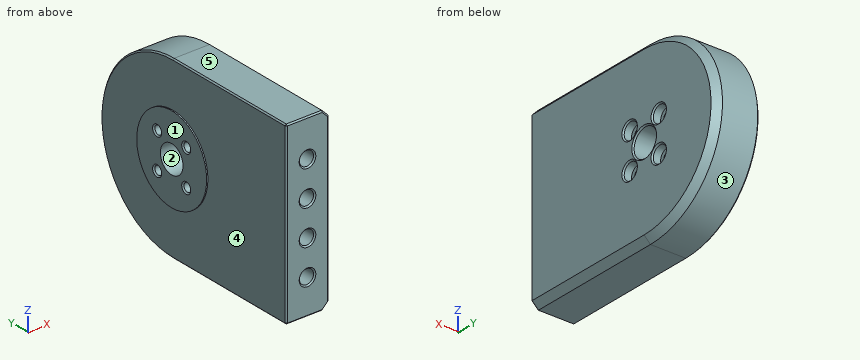
from build123d import *

# Parameters (mm, degrees)
SKETCH1_R                                           = 35
SKETCH1_R_2                                         = 5.5
SKETCH1_R_3                                         = 17
BOSS_EXTRUDE1_DEPTH                                 = 17
BOSS_EXTRUDE2_START                                 = -0.5
SKETCH1_3_R                                         = 17
SKETCH1_3_R_2                                       = 5.5
BOSS_EXTRUDE2_DEPTH                                 = 0.5
CBORE_FOR_M3_HEX_SOCKET_HEAD_CAP_SCREW1_D           = 3.4
CBORE_FOR_M3_HEX_SOCKET_HEAD_CAP_SCREW1_CBORE_D     = 6.5
CBORE_FOR_M3_HEX_SOCKET_HEAD_CAP_SCREW1_CBORE_DEPTH = 3.4
F_5_6_5_6_DIAMETER_HOLE1_D                          = 5.6
F_5_6_5_6_DIAMETER_HOLE1_DEPTH                      = 8
F_5_6_5_6_DIAMETER_HOLE1_TIP                        = 1.682409733
F_2_5MM_CHAMFER1_SIZE                               = 2.5
F_0_5MM_CHAMFER2_SIZE                               = 0.5


with BuildPart() as part:
    # Sketch1 → Boss-Extrude1 (new body)
    # profile 1 of 3: a face of its own
    with BuildSketch(Plane(origin=(0, 0, 0), x_dir=(0, 0, -1), z_dir=(1, 0, 0))):
        Circle(SKETCH1_R)
        Circle(SKETCH1_R_2, mode=Mode.SUBTRACT)
    # profile 2 of 3: a face of its own
    with BuildSketch(Plane(origin=(0, 0, 0), x_dir=(0, 0, -1), z_dir=(1, 0, 0))):
        with BuildLine():
            ThreePointArc((35, 0), (0, -35), (-35, 0))
            Line((-35, 0), (-35, -55))
            Line((-35, -55), (35, -55))
            Line((35, -55), (35, 0))
        make_face()
    # profile 3 of 3: a face of its own
    with BuildSketch(Plane(origin=(0, 0, 0), x_dir=(0, 0, -1), z_dir=(1, 0, 0))):
        Circle(SKETCH1_R_3)
        Circle(SKETCH1_R_2, mode=Mode.SUBTRACT)
    extrude(amount=BOSS_EXTRUDE1_DEPTH)

    # Sketch1<3> → Boss-Extrude2 (add)
    with BuildSketch(Plane(origin=(0, 0, 0), x_dir=(0, 0, -1), z_dir=(1, 0, 0)).offset(BOSS_EXTRUDE2_START)):
        Circle(SKETCH1_3_R)
        Circle(SKETCH1_3_R_2, mode=Mode.SUBTRACT)
    extrude(amount=BOSS_EXTRUDE2_DEPTH)

    # CBORE for M3 Hex Socket Head Cap Screw1 (through all)
    with Locations(Plane(origin=(17, 0, 0), x_dir=(0, 0, -1), z_dir=(1, 0, 0))):
        with Locations((-7.071067812, 7.071067812), (7.071067812, 7.071067812), (7.071067812, -7.071067812), (-7.071067812, -7.071067812)):
            CounterBoreHole(CBORE_FOR_M3_HEX_SOCKET_HEAD_CAP_SCREW1_D / 2, CBORE_FOR_M3_HEX_SOCKET_HEAD_CAP_SCREW1_CBORE_D / 2, CBORE_FOR_M3_HEX_SOCKET_HEAD_CAP_SCREW1_CBORE_DEPTH)

    # Ø5.6 (5.6) Diameter Hole1
    with Locations(Plane(origin=(0, -55, 0), x_dir=(-1, 0, 0), z_dir=(0, -1, 0))):
        with Locations((-8.5, -20.2), (-8.5, 21.2), (-8.5, 7.4), (-8.5, -6.4)):
            Hole(F_5_6_5_6_DIAMETER_HOLE1_D / 2, depth=F_5_6_5_6_DIAMETER_HOLE1_DEPTH)
            with Locations((0, 0, -(F_5_6_5_6_DIAMETER_HOLE1_DEPTH + F_5_6_5_6_DIAMETER_HOLE1_TIP / 2))):  # 118° drill point
                Cone(0, F_5_6_5_6_DIAMETER_HOLE1_D / 2, F_5_6_5_6_DIAMETER_HOLE1_TIP, mode=Mode.SUBTRACT)

    # 2,5mm Chamfer1
    f_2_5mm_chamfer1_edges = [part.edges().sort_by_distance(p)[0] for p in [
        (17, -27.5, 35),
        (17, -27.5, -35),
        (17, 35, 0),
    ]]
    chamfer(f_2_5mm_chamfer1_edges, length=F_2_5MM_CHAMFER1_SIZE)

    # 0,5mm Chamfer2
    f_0_5mm_chamfer2_edges = [part.edges().sort_by_distance(p)[0] for p in [
        (17, 0, 5.5),
        (17, 7.071067812, 10.321067812),
        (-0.5, 7.071067812, 5.371067812),
        (17, -7.071067812, 10.321067812),
        (-0.5, -7.071067812, 5.371067812),
        (17, -7.071067812, -3.821067812),
        (-0.5, -7.071067812, -8.771067812),
        (17, 7.071067812, -3.821067812),
        (-0.5, 7.071067812, -8.771067812),
        (5.7, -55, 20.2),
        (5.7, -55, 6.4),
        (5.7, -55, -7.4),
        (5.7, -55, -21.2),
        (0, -27.5, -35),
        (7.25, -55, -35),
        (17, -55, 0),
        (7.25, -55, 35),
        (0, -55, 0),
        (15.75, -55, 33.75),
        (15.75, -55, -33.75),
        (0, -27.5, 35),
        (0, 35, 0),
    ]]
    chamfer(f_0_5mm_chamfer2_edges, length=F_0_5MM_CHAMFER2_SIZE)


solid = part.part
Check sheet for the modelled part. Datum: model origin and axes. Units: mm. Face numbers are marked on the shaded views. A direction names the side the tool comes from. Give positions to 0.01 mm unless a question says otherwise; leave off trailing zeros. Write each loop counter-clockwise with the first axis right and the second up, starting at its lowest first coordinate (ties: lowest second). Pieces come first, ordered by that corner, then holes. Notation, with made-up numbers: (73, -18.75) -> (117, -18.75) arc R17 ccw to (117, 2.25) -> close; hole circle Ø5 at (-14.5, 58.5). An arc over 180 degrees is marked (long way). One line per item, written item: value. Start each with the question number.
Item 1: Draft check along Y on the marked faces 1, 2 and 3. Enter one of: +Y half, -Y half, draft (parallel to the pull), parting line (faces both ways), or undercut.
Item 2: Gauge pin test, flat ends, axial feed: pin 1 (9 mm diameter, centred on y = 0, z = 0, fed in from -X); pin 2 (5 mm diameter, centred on y = 7, z = 7, fed in from +X); pin 3 (2 mm diameter, centred on y = -13, z = -21, fed in from -X); pin 4 (3.5 mm diameter, centred on x = 8.5, z = 20.2, fed in from -Y). Record the tip position at first contact, or that the pin passes through.
Item 3: Material ranges on probe 1 along Z at (x, y) = (8.5, -51.5); probe 2 along Z at (x, y) = (4.5, 8.5); probe 3 along Z at (x, y) = (14.5, -4.5), recorded low to high. Write a range as from..to.
Item 4: Section check C-C on x = 9.5. State how many separate pieces and enclosed holes the cut face has, then the cut area to 3 significant figures.
Item 5: Tool access check on the marked faces 4 and 5. Record the directions out of +Z, -Z, +X, -X, +Y, -Y that give a thin tool (end or side, any length) a straight path to the whole face; none if there is none.
Item 6: Section check A-A on y = -39. Record the cut outline in (x, z), then the cut area to 3 significant figures.
Item 7: Section check B-B on x = 1.5. Record the cut outline in (y, z).
Results list:
1. face 1: draft
1. face 2: undercut
1. face 3: +Y half
2. pin 1: through
2. pin 2: x = 13.6
2. pin 3: x = 0
2. pin 4: y = -46.37
3. probe 1: -35..-24, -18.4..-10.2, -4.6..3.6, 9.2..17.4, 23..35
3. probe 2: -33.95..-7.99, -6.15..6.15, 7.99..33.95
3. probe 3: -35..-9.06, -5.08..-3.16, 3.16..5.08, 9.06..35
4. separate pieces: 1
4. enclosed holes: 5
4. area: 5,460 mm²
5. face 4: -X
5. face 5: +Z, +X, -X, +Y, -Y
6. outline: (0, -34.5) -> (0.5, -35) -> (14.5, -35) -> (17, -32.5) -> (17, 32.5) -> (14.5, 35) -> (0.5, 35) -> (0, 34.5) -> close
6. area: 1,180 mm²
7. outline: (-55, -34.5) -> (-54.5, -35) -> (0, -35) arc R35 ccw to (0, 35) -> (-54.5, 35) -> (-55, 34.5) -> close; hole circle Ø3.4 at (-7.07, -7.07); hole circle Ø3.4 at (-7.07, 7.07); hole circle Ø11 at (0, 0); hole circle Ø3.4 at (7.07, -7.07); hole circle Ø3.4 at (7.07, 7.07)
